Could you check a few things on this drawing? It's one solid part, dimensions in mm from its lowest x, y, z. A direction names the side the tool comes from. Round coordinates to 2 decimals unless told otherwise and drop trailing zeros. Write each loop counter-clockwise with the first axis right and the second up, starting at its lowest first coordinate (ties: lowest second). Pieces come first, ordered by that corner, then holes. Notation, with made-up numbers: (-38.5, -38.75) - (9.5, -38.75) arc R10 ccw to (9.5, -19.75) - close; hole circle Ø4 at (38, -31). An arc over 180 degrees is marked (long way). Write item = value, one per line. Start each with the question number.
Item 1: If I drill on line 1 along X through (y, z) = (1.7, 1.75) (1 decimal); line 2 along Z through (x, y) = (2.1, 0.5); line 3 along Y through (x, z) = (2.7, 0.75) (1 decimal), over which ranges is the centre line in solid material (lowest first)? Write a range as [from, to].
Item 2: If we section it at B-B (x = 2.25): Please give me the cut outline in (y, z) (1 decimal).
Item 3: Which directions (+Z, -Z, +X, -X, +Y, -Y) give clear straight access to the entire face, cutting with the end or side of a thin tool? Please do the marked faces 4, 5 and 6.
Item 4: If we section it at D-D (y = 0.5): Please give me the cut outline in (x, z).
Item 5: For P1, Ø1, axis at x = 2, z = 5.5, coming from the -Y side; P2, Ø3, axis at x = 0.5, z = 5.5, coming from the +Y side, each with a flat end and sliding along its axis, tell me the tip position at first contact or that it passes through.
Item 6: If we section it at C-C (z = 4): Please give me the cut outline in (x, y).
Item 7: Thinking about a two-plate mould opening in X: for the marked faces 1, 2 and 3, which applies, pulls with the +X half, pulls with the -X half, needs draft (parallel to the pull), parting line crosses it, or undercut?
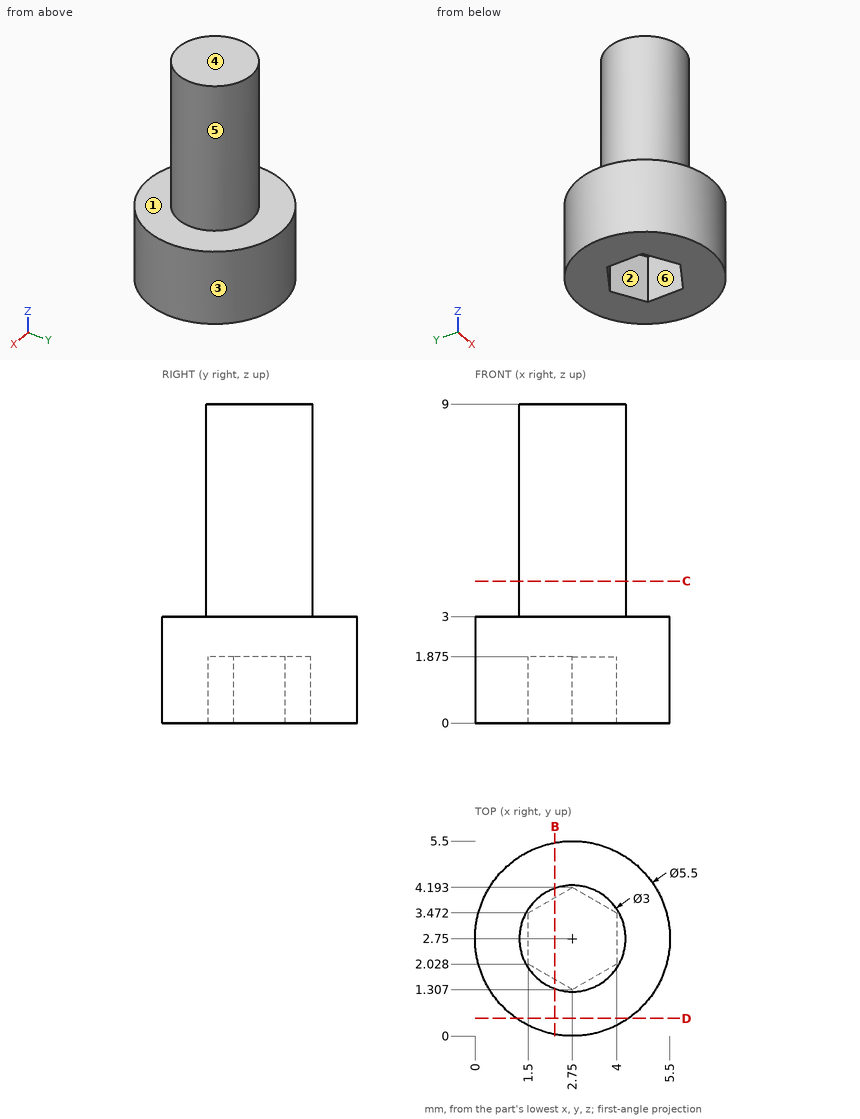
Reply:
q1.line_1 = [0.2, 2.1], [3.4, 5.3]
q1.line_2 = [0, 3]
q1.line_3 = [0, 1.3], [4.2, 5.5]
q2.outline = (0, 0) - (1.6, 0) - (1.6, 1.9) - (3.9, 1.9) - (3.9, 0) - (5.5, 0) - (5.5, 3) - (4.2, 3) - (4.2, 9) - (1.3, 9) - (1.3, 3) - (0, 3) - close
q3.face_4 = +Z, +X, -X, +Y, -Y
q3.face_5 = +Z
q3.face_6 = -Z
q4.outline = (1.17, 0) - (4.33, 0) - (4.33, 3) - (1.17, 3) - close
q5.P1 = 1.27
q5.P2 = 4.05
q6.outline = circle Ø3 at (2.75, 2.75)
q7.face_1 = needs draft
q7.face_2 = undercut
q7.face_3 = parting line crosses it
